Autodesk Fusion 360 part; units mm, degrees
sketch "Sketch1" plane through (0, 0, 0) normal (0, 1, 0) x (1, 0, 0)
  line L0 (0, 0) -> (-127.2538, 0)
  line L1 (-127.2538, 0) -> (-127.2538, -15.6248)
  line L2 (-127.2538, -15.6248) -> (0, 0)
  line L3 (-127.2538, 0) -> (-0.0202, 0)
  line L4 (0, 0) -> (-0.8531, 6.9478)
  line L5 (-0.8531, 6.9478) -> (-127.2538, -8.5722)
  line L6 (-127.2538, 6.9478) -> (-127.2538, -15.6248)
  line L7 (-127.2538, -8.5722) -> (-126.4008, -15.5201)
  line L8 (-0.8531, 6.9478) -> (-127.2538, 6.9478)
  line L9 (-0.8531, 6.9478) -> (0, 6.9478)
  line L10 (0, 6.9478) -> (0, 0)
  line L11 (-127.2538, 3.7478) -> (0, 3.7478)
  line L12 (-127.2538, 0.7478) -> (-56.2538, 0.7478)
  line L13 (-127.2538, 6.9478) -> (-128.8538, 6.9478)
  line L14 (0, 6.9478) -> (1.6, 6.9478)
  line L15 (1.6, 6.9478) -> (1.6, 0.1989)
  line L16 (-0.0202, 0) -> (1.6, 0.1989)
  line L17 (-128.8538, 6.9478) -> (-128.8538, -15.8213)
  line L18 (-127.2538, -15.6248) -> (-128.8538, -15.8213)
  line L19 (-0.6093, 4.9627) -> (-127.0101, -10.5573)
  line L20 (-87.2538, -3.6609) -> (-87.2538, 3.7478)
  line L21 (-56.2538, 3.7478) -> (-56.2538, 0.7478)
  line L22 (-127.2538, 3.7478) -> (-128.8538, 3.7478)
  circle A0 centre (-41.0275, 0) radius 2.1736
  dimension "d2" = 7
  dimension "d7" = 7
  dimension "d16" = 127.35
  dimension "d17" = 3.2
  dimension "d18" = 71
  dimension "d19" = 1.6
  dimension "d20" = 1.6
  dimension "d21" = 2
  dimension "d28" = 40
  dimension "d29" = 3
extrude "Extrude1" add sketch "Sketch1" along normal blind 362.2 contours L4 L10 L11 | L10 L14 L15 L16 | L4 L9 L10 L11 | L4 L5 L11 L19 | L5 L6 L8 L11 | L6 L13 L17 L22
sketch "Sketch2" plane through (0, 362.2, 0) normal (0, 1, 0) x (-1, 0, 0)
  line L0 (128.8538, -3.7478) -> (10.504, -3.7478)
  line L1 (0.0003, -0.0024) -> (-1.6, -0.1989)
  line L2 (-1.6, -0.1989) -> (-1.6, -6.9478)
  line L3 (-1.6, -6.9478) -> (128.8538, -6.9478)
  line L4 (128.8538, -6.9478) -> (128.8538, -3.7478)
  line L5 (0.0003, -0.0024) -> (-1.6, -0.1989)
  line L6 (-1.6, -0.1989) -> (-1.6, -6.9478)
  line L7 (-1.6, -6.9478) -> (128.8538, -6.9478)
  line L8 (128.8538, -6.9478) -> (128.8538, -3.7478)
  line L9 (128.8538, -3.7478) -> (0.0003, -0.0024)
  line L10 (0.6093, -4.9627) -> (0.0003, -0.0024)
  line L11 (10.504, -3.7478) -> (0.6093, -4.9627)
sketch "Sketch3" plane through (0, 0, -6.9478) normal (0, 0, -1) x (1, 0, 0)
  line L0 (1.6, 0) -> (-128.8538, 0)
  line L1 (-128.8538, 0) -> (-128.8538, -362.2)
  line L2 (-128.8538, -362.2) -> (1.6, -362.2)
  line L3 (1.6, -362.2) -> (1.6, 0)
  line L4 (1.6, -362.2) -> (-128.8538, -362.2)
  line L5 (-128.8538, -362.2) -> (-128.8538, 0)
  line L6 (-128.8538, 0) -> (1.6, 0)
  line L7 (1.6, 0) -> (1.6, -362.2)
  circle A0 centre (-124.0538, -3.2) radius 1.55
  circle A1 centre (-3.2, -3.2) radius 1.55
  circle A2 centre (-3.2, -359) radius 1.55
  circle A3 centre (-124.0538, -359) radius 1.55
  line L8 (-48.641, 0) -> (-48.641, -362.2)
  line L9 (-128.8538, -181.1) -> (1.6, -181.1)
  line L10 (-48.641, -268.45) -> (1.6, -268.45)
  circle A4 centre (-48.641, -268.45) radius 1.55
  circle A5 centre (-48.641, -348.187) radius 1.55
  line L11 (-128.8538, -362.2) -> (-0.0003, -362.2)
  circle A6 centre (-48.641, -188.713) radius 1.55
  circle A7 centre (-48.641, -173.487) radius 1.55
  line L12 (-48.641, -93.75) -> (1.6, -93.75)
  circle A8 centre (-48.641, -93.75) radius 1.55
  circle A9 centre (-48.641, -14.013) radius 1.55
  line L13 (-127.2538, 0) -> (0, 0)
  dimension "d30" = 3.1
  dimension "d31" = 3.2
  dimension "d32" = 4.8
  dimension "d33" = 3.1
  dimension "d34" = 4.8
  dimension "d35" = 3.2
  dimension "d36" = 3.1
  dimension "d37" = 4.8
  dimension "d38" = 3.2
  dimension "d39" = 3.1
  dimension "d40" = 4.8
  dimension "d41" = 3.2
  dimension "d43" = 181.1
  dimension "d44" = 87.35
  dimension "d45" = 50.241
  dimension "d46" = 3.1
  dimension "d47" = 3.1
  dimension "d48" = 14.013
  dimension "d49" = 3.1
  dimension "d50" = 7.613
  dimension "d51" = 3.1
  dimension "d52" = 7.613
  dimension "d53" = 87.35
  dimension "d54" = 3.1
  dimension "d55" = 3.1
  dimension "d56" = 14.013
hole "Hole1" at (-48.641, 173.487, -6.9478) direction (0, 0, 1) diameter 3.1 end through all
hole "Hole2" at (-48.641, 348.187, -6.9478) direction (0, 0, 1) diameter 3.1 end through all
hole "Hole3" at (-48.641, 268.45, -6.9478) direction (0, 0, 1) diameter 3.1 end through all
hole "Hole4" at (-48.641, 188.713, -6.9478) direction (0, 0, 1) diameter 3.1 end through all
hole "Hole5" at (-48.641, 93.75, -6.9478) direction (0, 0, 1) diameter 3.1 end through all
hole "Hole6" at (-48.641, 14.013, -6.9478) direction (0, 0, 1) diameter 3.1 end through all
hole "Hole7" at (-3.2, 359, -6.9478) direction (0, 0, 1) diameter 3.1 end through all
hole "Hole8" at (-124.0538, 359, -6.9478) direction (0, 0, 1) diameter 3.1 end through all
hole "Hole9" at (-3.2, 3.2, -6.9478) direction (0, 0, 1) diameter 3.1 end through all
hole "Hole10" at (-124.0538, 3.2, -6.9478) direction (0, 0, 1) diameter 3.1 end through all
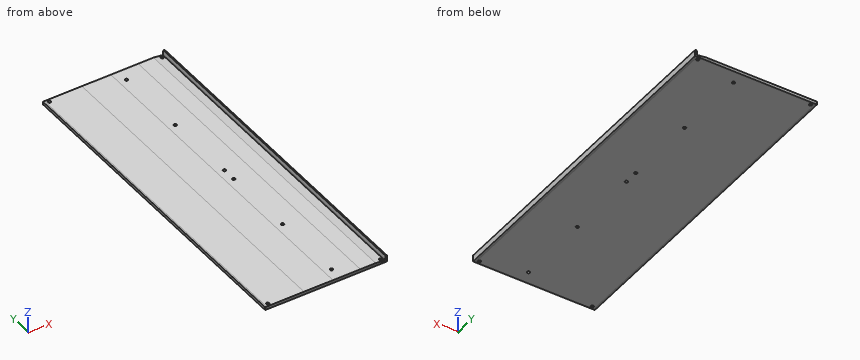
Geometry: final body of the model. Coordinates: model frame, mm. Round coordinates to 2 decimals unless told otherwise and drop trailing zeros. Write each loop counter-clockwise with the first axis right and the second up, starting at its lowest first coordinate (ties: lowest second). Pieces come first, ordered by that corner, then holes. Notation, with made-up numbers: M 8.5,0 L 28.5,0 A20 cw 28.5,18 Z; hole C 32.5,-36 d6. An arc over 180 degrees is marked long. Answer in a Markdown table with one row per item. Add a question column.
(1) Cut plane A-A, the plane y = 300. Return the cut outline in (x, z).
(2) Cut plane C-C, the plane z = -1.25. Return the cut outline in (x, y), then the cut area to 3 significant figures.
(3) Contact query for flat-ended pins moving along their axis: pin 1 (25 mm diameter, centred on x = -77, y = 152, fed in from +Z); pin 2 (1.9 mm diameter, centred on x = -3.2, y = 359, fed in from -Z). Output: stop coordinate, or through.
(4) Ray query, L1, parallel to Y at x = -3.2, z = -5.7; L2, parallel to X at y = 3.2, z = -4.7; L3, parallel to X at y = 3.2, z = -5.25. Return the intervals inside material, ascending.
(5) Cut plane B-B, the plane x = -16. Return the cut outline in (y, z), then the cut area to 3 significant figures.
Established:
| question | item | result |
|---|---|---|
| 1 | outline | M -128.85,-6.95 L 1.6,-6.95 L 1.6,-0.2 L 0,0 L -0.61,-4.96 L -10.5,-3.75 L -128.85,-3.75 Z |
| 2 | outline | M -0.15,0 L 1.6,0 L 1.6,362.2 L -0.15,362.2 Z |
| 2 | area | 635 mm² |
| 3 | pin 1 | z = -3.75 |
| 3 | pin 2 | through |
| 4 | L1 | 0 to 1.65, 4.75 to 357.45, 360.55 to 362.2 |
| 4 | L2 | -128.85 to -125.6, -122.5 to -4.75, -0.58 to 1.6 |
| 4 | L3 | -128.85 to -125.6, -122.5 to -4.75, -1.65 to 1.6 |
| 5 | outline | M 0,-6.95 L 362.2,-6.95 L 362.2,-3.75 L 0,-3.75 Z |
| 5 | area | 1,160 mm² |
